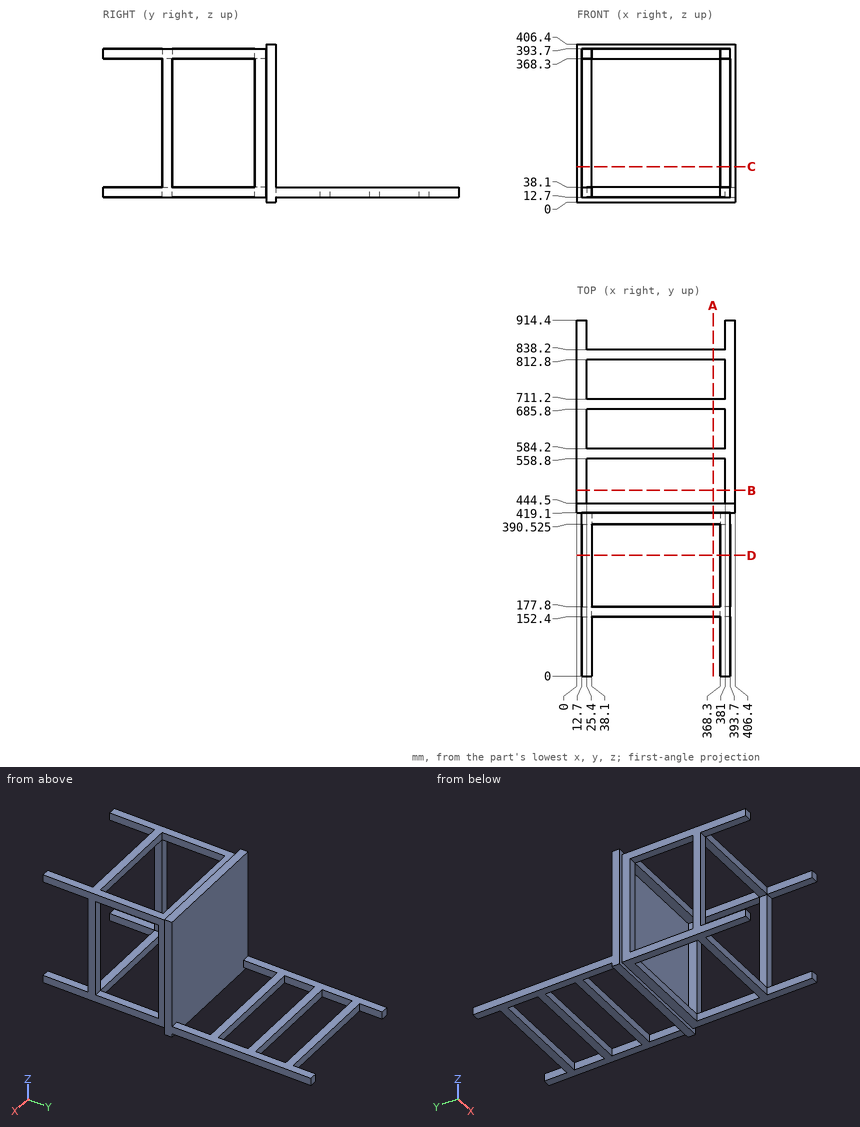
Design review of the part shown in the three views and the two pictorial views. Dimensions are in mm from the part's minimum x, y and z. Round coordinates to 2 decimals unless told otherwise and drop trailing zeros. Loops run counter-clockwise (first coordinate to the right, second up) from the corner with the lowest first, then second, coordinate; pieces in that order, holes last. Notation, with made-up numbers: M 88.5,3 L 104.5,3 A17 cw 104.5,15 Z; hole C 4,60 d7. An arc over 180 degrees is marked long. Answer as a JSON object with one key per item and string values.
Item 1: For line 1 along X through (y, z) = (165.5, 64.5); line 2 along Y through (x, z) = (99, 390) (3 decimals), list the stretches that pass through material, from the lowest coordinate up.
Check sheet entries:
{"line 1": "12.7 to 38.1, 368.3 to 393.7", "line 2": "152.4 to 177.8, 390.525 to 444.5"}
Item 2: We need section C-C, the plane z = 91. State the section outline as (x, y) points (3 decimals).
Check sheet entries:
{"outline": "M 0,419.1 L 12.7,419.1 L 12.7,390.525 L 38.1,390.525 L 38.1,419.1 L 368.3,419.1 L 368.3,390.525 L 393.7,390.525 L 393.7,419.1 L 406.4,419.1 L 406.4,444.5 L 0,444.5 Z; M 12.7,152.4 L 38.1,152.4 L 38.1,177.8 L 12.7,177.8 Z; M 368.3,152.4 L 393.7,152.4 L 393.7,177.8 L 368.3,177.8 Z"}
Item 3: We need section D-D, the plane y = 310. State the section outline as (x, z) points.
Check sheet entries:
{"outline": "M 12.7,12.7 L 38.1,12.7 L 38.1,38.1 L 12.7,38.1 Z; M 12.7,368.3 L 38.1,368.3 L 38.1,393.7 L 12.7,393.7 Z; M 368.3,12.7 L 393.7,12.7 L 393.7,38.1 L 368.3,38.1 Z; M 368.3,368.3 L 393.7,368.3 L 393.7,393.7 L 368.3,393.7 Z"}
Item 4: We need section A-A, the plane x = 350.5. State how many separate pieces and enclosed holes the cut face has, and give its area (3 significant figures).
Check sheet entries:
{"separate pieces": "6", "enclosed holes": "0", "area": "15,000 mm2"}
Item 5: Clearance check with flat-ended pins moving along their axes: P1, Ø12.5, axis at x = 31, y = 287, coming from the -Z side; P2, Ø7.5, axis at x = 27.5, y = 59.5, coming from the +Z side; P3, Ø3, axis at x = 120, z = 155.5, coming from the -Y side. State where each tip first meets the part, or that it passes through.
Check sheet entries:
{"P1": "z = 12.7", "P2": "z = 393.7", "P3": "y = 419.1"}
Item 6: We need section B-B, the plane y = 477. State the section outline as (x, z) points, and give its area (3 significant figures).
Check sheet entries:
{"outline": "M 0,12.7 L 25.4,12.7 L 25.4,38.1 L 0,38.1 Z; M 381,12.7 L 406.4,12.7 L 406.4,38.1 L 381,38.1 Z", "area": "1,290 mm2"}
